Part model, mm, in its own coordinate system. Face numbers are marked on the shaded views. Coordinates: 2 decimals unless noted, no trailing zeros. Write each loop counter-clockwise with the first axis right and the second up, starting at its lowest first coordinate (ties: lowest second). Pieces come first, ordered by that corner, then holes. Notation, with made-up numbers: M 38,40 L 57,40 A26 ccw 57,54 Z; hole C 11,7 d5. An arc over 180 degrees is marked long. Use a Markdown table: item, result. Add a question column.
Q1. Pin check, flat tips, straight feed: pin 1 Ø1.5 at (y, z) = (-0.5, 2.5) entering from -X; pin 2 Ø1.8 at (x, z) = (-3.5, 0) entering from -Y. Stop position of each tip, or through.
Q2. Slice it at D-D on z = 0.25. Write the cut outline in (x, y), then the cut area to 3 significant figures.
Q3. Slice it at A-A on z = -1. Write the cut outline in (x, y), then the cut area to 3 significant figures.
Q4. Slice it at C-C on y = 0.45. Count the separate pieces of the cut face and the enclosed holes in it, then the cut area to 3 significant figures.
Q5. Wall check: L1, parallel to X at y = 0.7, z = 1.25; L2, parallel to X at y = 0.85, z = 0.5; L3, parallel to Z at x = -4, y = -1.15. Give the ranges that are in metal, low to high. Write a range as from..to.
Q6. Slice it at B-B on x = 3.75. Write the cut outline in (y, z).
Q7. Mould opens along Z. For the marked faces 1, 2, 3 and 4 say: released by +Z, released by -Z, zero draft, split by the parting line, or undercut.
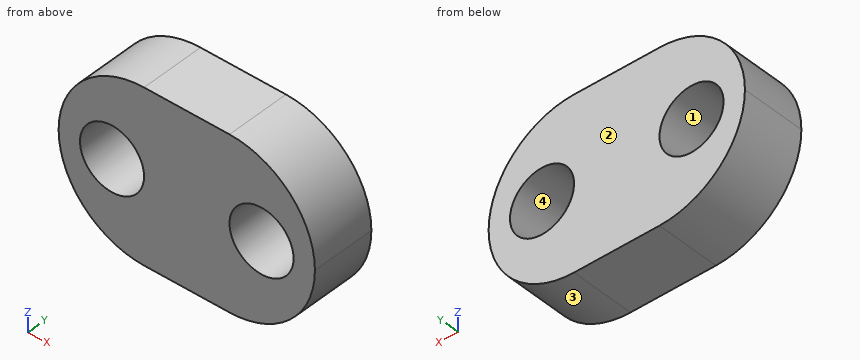
from build123d import *

# Parameters (mm, degrees)
F0_W     = 12
F0_H     = 3
F1_DEPTH = 4
F2_R     = 1.5
F3_DEPTH = 25
F4_R     = 3.99999


# Not quite as in the source:
# - a fillet or chamfer is up to 0.001 mm smaller than in the source, because OpenCascade refuses the exact size


with BuildPart() as f1:
    # F0 (on Top) → F1 (new body, symmetric)
    with BuildSketch(Plane.XY):
        Rectangle(F0_W, F0_H)
    extrude(amount=F1_DEPTH, both=True)

    # F2 (on face) → F3 (cut)
    with BuildSketch(Plane.XZ.offset(1.5)):
        with Locations((-3.5, 0)):
            Circle(F2_R)
        with Locations((3.5, 0)):
            Circle(F2_R)
    extrude(amount=-F3_DEPTH, mode=Mode.SUBTRACT)

    # F4 (radius 4 in the source; OpenCascade refuses exactly that, so slightly less here)
    f4_edges = [f1.edges().sort_by_distance(p)[0] for p in [
        (-6, 0, 4),
        (-6, 0, -4),
        (6, 0, 4),
        (6, 0, -4),
    ]]
    fillet(f4_edges, radius=F4_R)


solid = f1.part
Recorded:
| question | item | result |
|---|---|---|
| 1 | pin 1 | x = -5.6 |
| 1 | pin 2 | through |
| 2 | outline | M -5.99,-1.5 L -4.98,-1.5 L -4.98,1.5 L -5.99,1.5 Z; M -2.02,-1.5 L 2.02,-1.5 L 2.02,1.5 L -2.02,1.5 Z; M 4.98,-1.5 L 5.99,-1.5 L 5.99,1.5 L 4.98,1.5 Z |
| 2 | area | 18.2 mm² |
| 3 | outline | M -5.87,-1.5 L -4.62,-1.5 L -4.62,1.5 L -5.87,1.5 Z; M -2.38,-1.5 L 2.38,-1.5 L 2.38,1.5 L -2.38,1.5 Z; M 4.62,-1.5 L 5.87,-1.5 L 5.87,1.5 L 4.62,1.5 Z |
| 3 | area | 21.8 mm² |
| 4 | separate pieces | 1 |
| 4 | enclosed holes | 2 |
| 4 | area | 68.1 mm² |
| 5 | L1 | -5.8..-4.33, -2.67..2.67, 4.33..5.8 |
| 5 | L2 | -5.97..-4.91, -2.09..2.09, 4.91..5.97 |
| 5 | L3 | -3.46..-1.41, 1.41..3.46 |
| 6 | outline | M -1.5,-3.6 L 1.5,-3.6 L 1.5,-1.48 L -1.5,-1.48 Z; M -1.5,1.48 L 1.5,1.48 L 1.5,3.6 L -1.5,3.6 Z |
| 7 | face 1 | undercut |
| 7 | face 2 | zero draft |
| 7 | face 3 | released by -Z |
| 7 | face 4 | undercut |
